The listing builds one solid part. Answer for the finished solid, in the listing's coordinates (mm). Face numbers are marked on the shaded views. Coordinates: 2 decimals unless noted, no trailing zeros. Order: outer loops, then holes, each group sorted by start corner. A loop starts at its lowest first (then second) coordinate and runs counter-clockwise, first axis right, second up. Notation, with made-up numbers: (23, 61.25) -> (75, 61.25) arc R25 cw to (75, 86.25) -> close; hole circle Ø5 at (77.5, -15). An arc over 180 degrees is marked (long way). Write item = value, one per line.
from build123d import *

# Parameters (mm, degrees)
SKETCH_1_R                       = 17.5
EXTRUDE_1_DEPTH                  = 1
SKETCH_2_R                       = 15.915
EXTRUDE_2_DEPTH                  = 11
SKETCH_3_R                       = 17.5
EXTRUDE_3_DEPTH                  = 1
SKETCH_4_R                       = 11.5
EXTRUDE_4_DEPTH                  = 12
SKETCH_5_R                       = 4
CUT_EXTRUDE_1_DEPTH              = 36.178118199
HOLE_WIZARD_M4_1_REACH           = 40.674
HOLE_WIZARD_M4_1_BORE_R          = 1.65
HOLE_WIZARD_M4_1_ON_FACE_2_REACH = 40.693
HOLE_WIZARD_M4_1_BORE_2_R        = 1.65


with BuildPart() as part:
    # 草图1 → 凸台-拉伸1 (new body)
    with BuildSketch(Plane(origin=(0, 0, 0), x_dir=(1, 0, 0), z_dir=(0, 1, 0))):
        with Locations(Location((0, 0, 0), (0, 0, 270))):
            Circle(SKETCH_1_R)
    extrude(amount=EXTRUDE_1_DEPTH)

    # 草图2 → 凸台-拉伸2 (add)
    with BuildSketch(Plane(origin=(0, 1, 0), x_dir=(1, 0, 0), z_dir=(0, 1, 0))):
        with Locations(Location((0, 0, 0), (0, 0, 270))):
            Circle(SKETCH_2_R)
    extrude(amount=EXTRUDE_2_DEPTH)

    # 草图3 → 凸台-拉伸3 (add)
    with BuildSketch(Plane(origin=(0, 12, 0), x_dir=(1, 0, 0), z_dir=(0, 1, 0))):
        with Locations(Location((0, 0, 0), (0, 0, 270))):
            Circle(SKETCH_3_R)
    extrude(amount=EXTRUDE_3_DEPTH)

    # 草图4 → 凸台-拉伸4 (add)
    with BuildSketch(Plane(origin=(0, 13, 0), x_dir=(1, 0, 0), z_dir=(0, 1, 0))):
        with Locations(Location((0, 0, 0), (0, 0, 270))):
            Circle(SKETCH_4_R)
    extrude(amount=EXTRUDE_4_DEPTH)

    # 草图5 → 切除-拉伸1 (cut, through all)
    with BuildSketch(Plane(origin=(0, 25, 0), x_dir=(1, 0, 0), z_dir=(0, 1, 0))):
        with Locations(Location((0, 0, 0), (0, 0, 270))):
            Circle(SKETCH_5_R)
    extrude(amount=-CUT_EXTRUDE_1_DEPTH, mode=Mode.SUBTRACT)

    # M4 螺纹孔1 bore (on position points) → M4 螺纹孔1 (cut, up to next)
    with BuildSketch(Plane(origin=(11.499382171, 18.555582634, -0.119204379), x_dir=(0.010365598164, 0, 0.999946275744), z_dir=(0.999946275744, 0, -0.010365598164)), mode=Mode.PRIVATE) as hole_wizard_m4_1_sk1:
        Circle(HOLE_WIZARD_M4_1_BORE_R)
    hole_wizard_m4_1_tool1 = extrude(hole_wizard_m4_1_sk1.sketch, amount=-HOLE_WIZARD_M4_1_REACH, mode=Mode.PRIVATE) & part.part
    add(hole_wizard_m4_1_tool1.solids().sort_by_distance((11.499382, 18.555583, -0.119204))[0], mode=Mode.SUBTRACT)

    # M4 螺纹孔1 bore 2 (on position points) → M4 螺纹孔1 on face 2 (cut, up to next)
    with BuildSketch(Plane(origin=(0.03684499, 18.671535984, 11.499940976), x_dir=(0.99999486718, 0, -0.003203999574), z_dir=(0.003203999574, 0, 0.99999486718)), mode=Mode.PRIVATE) as hole_wizard_m4_1_on_face_2_sk1:
        Circle(HOLE_WIZARD_M4_1_BORE_2_R)
    hole_wizard_m4_1_on_face_2_tool1 = extrude(hole_wizard_m4_1_on_face_2_sk1.sketch, amount=-HOLE_WIZARD_M4_1_ON_FACE_2_REACH, mode=Mode.PRIVATE) & part.part
    add(hole_wizard_m4_1_on_face_2_tool1.solids().sort_by_distance((0.036845, 18.671536, 11.499941))[0], mode=Mode.SUBTRACT)


solid = part.part
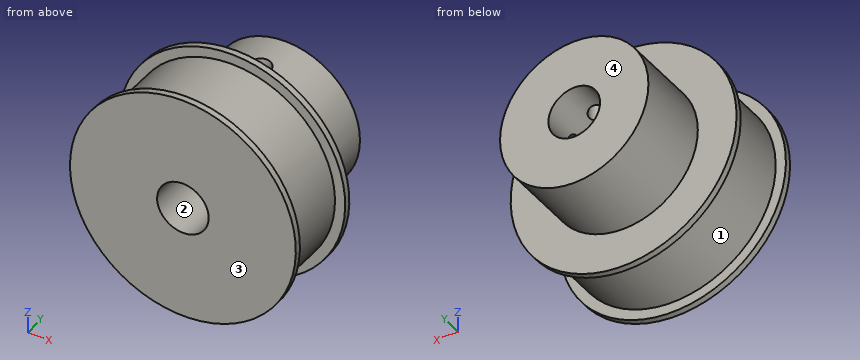
Q1. The mould has two halves that part along Y. Classify the marked faces 1, 2, 3 and 4: released by +Y, released by -Y, zero draft, split by the parting line, or undercut.
The answers:
face_1 = undercut
face_2 = zero draft
face_3 = released by -Y
face_4 = released by +Y
Q2. Section B-B, the plane x = -12 is taken. Give the vertices of the cut face in (y, z).
The answers:
outline = (0, -12.74) -> (1, -12.74) -> (1, -10.45) -> (12, -10.45) -> (12, -12.74) -> (13, -12.74) -> (13, 12.74) -> (12, 12.74) -> (12, 10.45) -> (1, 10.45) -> (1, 12.74) -> (0, 12.74) -> close
Q3. Section A-A, the plane y = 18 is taken. Give the vertices of the cut face in (x, z), plus the area to 3 significant figures.
The answers:
outline = (-1.5, 3.71) -> (-1.47, 11.41) arc R11.5 ccw (long way) to (11.38, -1.67) -> (3.67, -1.59) arc R4 cw (long way) to start; (1.52, 3.7) arc R4 cw to (3.7, 1.52) -> (11.41, 1.44) arc R11.5 ccw to (1.54, 11.4) -> close
area = 319 mm2
Q4. Section C-C, the plane z = -15 is taken. Give the vertices of the cut face in (x, y), plus the area to 3 significant figures.
The answers:
outline = (-9.01, 0) -> (9.01, 0) -> (9.01, 1) -> (5.32, 1) -> (5.32, 12) -> (9.01, 12) -> (9.01, 13) -> (-9.01, 13) -> (-9.01, 12) -> (-5.32, 12) -> (-5.32, 1) -> (-9.01, 1) -> close
area = 153 mm2
Q5. Section D-D, the plane y = 10.75 is taken. Give the vertices of the cut face in (x, z) (3 decimals).
The answers:
outline = circle Ø31.83 at (0, 0); hole circle Ø8 at (0, 0)
Q6. Find the intervals of material crossed by line 1 along Y through (x, z) = (12, -11.5); line 2 along X through (y, z) = (14, 0); line 3 along X through (y, z) = (7.75, 0) (3 decimals), in increasing order.
The answers:
line_1 = 0 to 1, 12 to 13
line_2 = -11.5 to -4, 4 to 11.5
line_3 = -15.915 to -4, 4 to 15.915
Q7. Each of these flat-tipped pins is pushed along its axis until it touches: pin 1 Ø12 at (x, y) = (11.5, 22.5) entering from -Z; pin 2 Ø1.5 at (x, y) = (12.5, 10) entering from -Z; pin 3 Ø4 at (x, y) = (7.5, 10.5) entering from +Z; pin 4 Ø17.5 at (x, z) = (1.5, -2) entering from +Y. Where does it stop, or does it pass through?
The answers:
pin_1 = -10.1
pin_2 = -10.73
pin_3 = 16.37
pin_4 = 25
